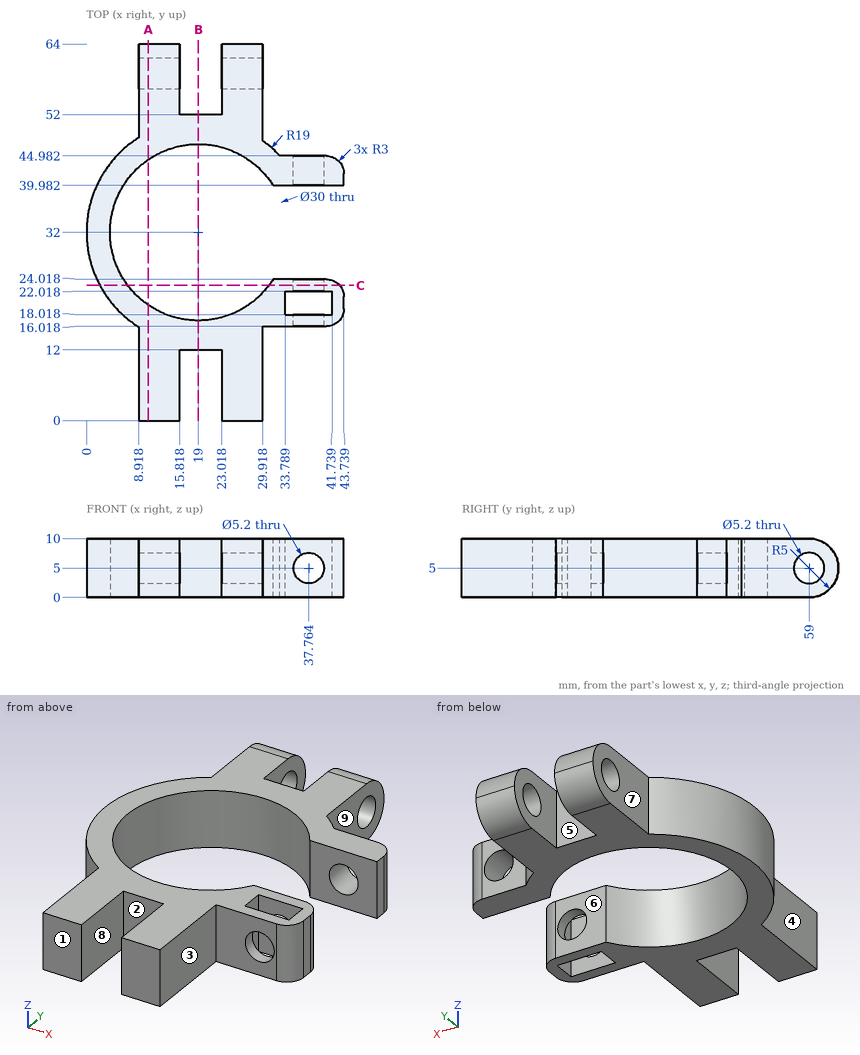
Verification items for this drawing (mm, ordinates from the low corner). A direction names the side the tool comes from. Round coordinates to 2 decimals unless told otherwise and drop trailing zeros. Order: outer loops, then holes, each group sorted by start corner. A loop starts at its lowest first (then second) coordinate and runs counter-clockwise, first axis right, second up. Notation, with made-up numbers: (12.5, -38) -> (71.5, -38) arc R16 ccw to (71.5, -32) -> close; hole circle Ø11 at (72, -26). An arc over 180 degrees is marked (long way). Use one line per item in the form item = value.
1. Scan lines: line 1 along Y through (x, z) = (35, 9.25); line 2 along Z through (x, y) = (24, 59); line 3 along Y through (x, z) = (28, 4). Record each from-to range of solid material in increasing order. Write a range as from..to.
Working result:
line_1 = 16.02..18.02, 22.02..24.02, 39.98..44.98
line_2 = 0..2.4, 7.6..10
line_3 = 0..20, 44..56.6, 61.4..63.9
2. Set-up check for the marked faces 5, 6, 7, 8 and 9: record each of +Z, -Z, +X, -X, +Y, -Y from which the full face is reachable in a straight line by a thin tool's end or side.
Working result:
face_5 = +Z, -Z, +Y
face_6 = +Z, -Z, +X
face_7 = +Z, -Z, -X, +Y
face_8 = +Z, -Z, -Y
face_9 = +Z, -Z, +X, +Y
3. Cross-section at C-C, the plane y = 23. Enter the section's corners in (x, z), plus the area to 3 significant figures.
Working result:
outline = (2.27, 0) -> (7, 0) -> (7, 10) -> (2.27, 10) -> close; (31, 0) -> (42.99, 0) -> (42.99, 10) -> (31, 10) -> close; hole circle Ø5.2 at (37.76, 5)
area = 146 mm^2
4. Cross-section at B-B, the plane x = 19. Enter the section's corners in (y, z), plus the area to 4 significant figures.
Working result:
outline = (12, 0) -> (17, 0) -> (17, 10) -> (12, 10) -> close; (47, 0) -> (52, 0) -> (52, 10) -> (47, 10) -> close
area = 100.0 mm^2
5. Go/stop test with flat-tipped pins: pin 1 (1.5 mm diameter, centred on y = 9, z = 9, fed in from -X); pin 2 (2.5 mm diameter, centred on x = 35.5, z = 6.5, fed in from +Y); pin 3 (5 mm diameter, centred on x = 39.5, z = 3.5, fed in from -Y). Record where each tip stops, or that it passes through.
Working result:
pin_1 = 8.92
pin_2 = 44.98
pin_3 = 16.02
6. Cross-section at A-A, the plane x = 10.5. Enter the section's corners in (y, z).
Working result:
outline = (0, 0) -> (19.64, 0) -> (19.64, 10) -> (0, 10) -> close; (44.36, 0) -> (59, 0) arc R5 ccw to (59, 10) -> (44.36, 10) -> close; hole circle Ø5.2 at (59, 5)
7. Mould release check, pull along X, two halves, no side actions. Record for the marked faces 1, 2, 3 and 4: pulls with the +X half, pulls with the -X half, needs draft (parallel to the pull), parting line crosses it, or undercut.
Working result:
face_1 = needs draft
face_2 = undercut
face_3 = pulls with the +X half
face_4 = pulls with the -X half
